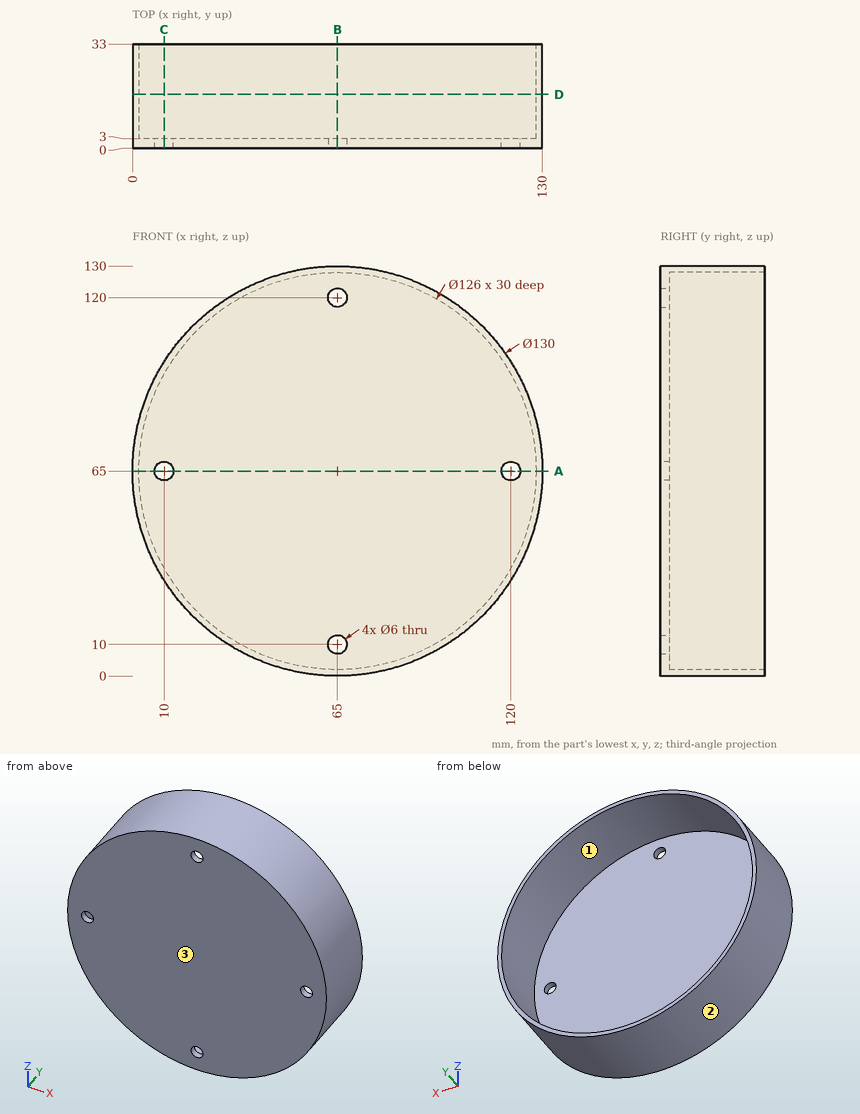
For this review, use the dimensioned drawing (mm, ordinates from the lowest corner) and the shaded views. Round coordinates to 2 decimals unless told otherwise and drop trailing zeros. Write each loop counter-clockwise with the first axis right and the second up, starting at its lowest first coordinate (ties: lowest second). Pieces come first, ordered by that corner, then holes. Notation, with made-up numbers: (88.5, 14.25) -> (99.5, 14.25) arc R9 cw to (99.5, 26.25) -> close; hole circle Ø1 at (-36, 16.25). An arc over 180 degrees is marked (long way). Answer in a Markdown table with one row per item.
Q1. Take a section at B-B, the plane x = 65. State the section outline as (y, z) points.
The answers:
| item | result |
|---|---|
| outline | (0, 0) -> (33, 0) -> (33, 2) -> (3, 2) -> (3, 7) -> (0, 7) -> close; (0, 13) -> (3, 13) -> (3, 117) -> (0, 117) -> close; (0, 123) -> (3, 123) -> (3, 128) -> (33, 128) -> (33, 130) -> (0, 130) -> close |
Q2. Clearance check with flat-ended pins moving along their axes: pin 1 Ø10 at (x, y) = (42, 10.5) entering from -Z; pin 2 Ø8 at (x, z) = (65, 10) entering from +Y; pin 3 Ø1.5 at (y, z) = (10.5, 96) entering from +X. State where each tip first meets the part, or that it passes through.
The answers:
| item | result |
|---|---|
| pin 1 | z = 2.54 |
| pin 2 | y = 3 |
| pin 3 | x = 122.53 |
Q3. Take a section at A-A, the plane z = 65. State the section outline as (x, y) points, then the cut area to 3 significant figures.
The answers:
| item | result |
|---|---|
| outline | (0, 0) -> (7, 0) -> (7, 3) -> (2, 3) -> (2, 33) -> (0, 33) -> close; (13, 0) -> (117, 0) -> (117, 3) -> (13, 3) -> close; (123, 0) -> (130, 0) -> (130, 33) -> (128, 33) -> (128, 3) -> (123, 3) -> close |
| area | 474 mm² |
Q4. To check wall thickness, follow L1, parallel to Z at x = 65, y = 0.8; L2, parallel to Z at x = 65, y = 17. State the ranges of each line that lie inside material, in increasing order. Write a range as [from, to].
The answers:
| item | result |
|---|---|
| L1 | [0, 7], [13, 117], [123, 130] |
| L2 | [0, 2], [128, 130] |
Q5. Take a section at D-D, the plane y = 17. State the section outline as (x, z) points.
The answers:
| item | result |
|---|---|
| outline | circle Ø130 at (65, 65); hole circle Ø126 at (65, 65) |
Q6. Draft analysis for pull direction Z (two halves, no side actions). For the marked faces 1, 2 and 3, state which applies: +Z half, -Z half, draft (parallel to the pull), parting line (faces both ways), or undercut.
The answers:
| item | result |
|---|---|
| face 1 | undercut |
| face 2 | parting line |
| face 3 | draft |
Q7. Take a section at C-C, the plane x = 10. State the section outline as (y, z) points, then the cut area to 3 significant figures.
The answers:
| item | result |
|---|---|
| outline | (0, 30.36) -> (33, 30.36) -> (33, 34.28) -> (3, 34.28) -> (3, 62) -> (0, 62) -> close; (0, 68) -> (3, 68) -> (3, 95.72) -> (33, 95.72) -> (33, 99.64) -> (0, 99.64) -> close |
| area | 425 mm² |
